from build123d import *

# Parameters (mm, degrees)
SUPPORT_BALISE_W                           = 20
SUPPORT_BALISE_H                           = 350
SUPPORT_BALISE_BOSSAGE_DEPTH               = 80
ESQUISSE3_W                                = 80
ESQUISSE3_H                                = 80
SUPPORT_CHEVAL_ENLEVEMENT_DE_MATIERE_DEPTH = 10
ESQUISSE8_W                                = 10
ESQUISSE8_H                                = 70
SUPPORT_CHEVAL_DEPTH                       = 80
VIS_REACH                                  = 376.466
SERRAGE_VIS_R                              = 2.5
VIS_DIRECTION_2_DEPTH                      = 375.466286867
ENL_V_MAT_EXTRU_5_DEPTH                    = 20
POUR_IMPRESSION_R                          = 15
FIXATION_POUR_ASSEMBLAGE_R                 = 2
VIS_POUR_ASSEMBLAGE_DEPTH                  = 20
ENL_V_MAT_EXTRU_6_DEPTH                    = 378.359245282
ENL_V_MAT_EXTRU_6_DEPTH_BACK               = 378.359245282
PARTIE_HAUTE_W                             = 433.052929697
PARTIE_HAUTE_H                             = 227.316532038


with BuildPart() as part:
    # Support Balise → Support balise bossage (new body)
    with BuildSketch(Plane.XY):
        with Locations((10, 175)):
            Rectangle(SUPPORT_BALISE_W, SUPPORT_BALISE_H)
    extrude(amount=SUPPORT_BALISE_BOSSAGE_DEPTH)

    # Esquisse3 → Support Cheval enlevement de matiere (add)
    with BuildSketch(Plane(origin=(0, 350, 0), x_dir=(1, 0, 0), z_dir=(0, 1, 0))):
        with Locations((-20, -40)):
            Rectangle(ESQUISSE3_W, ESQUISSE3_H)
    extrude(amount=SUPPORT_CHEVAL_ENLEVEMENT_DE_MATIERE_DEPTH)

    # Esquisse8 → Support Cheval (cut)
    with BuildSketch(Plane.XY.offset(80)):
        with Locations((10, 35)):
            Rectangle(ESQUISSE8_W, ESQUISSE8_H)
    extrude(amount=-SUPPORT_CHEVAL_DEPTH, mode=Mode.SUBTRACT)

    # Vis: up to this face of the body (flat: up to its plane)
    vis_end = Plane(part.part.faces().sort_by_distance((0, 175, 40))[0])
    # Serrage vis → Vis (cut, up to the picked face)
    with BuildSketch(Plane(origin=(5, 0, 0), x_dir=(0, 0, -1), z_dir=(1, 0, 0)), mode=Mode.PRIVATE) as vis_sk1:
        with Locations((-70, 11.284552026)):
            Circle(SERRAGE_VIS_R)
    vis_tool1 = split(extrude(vis_sk1.sketch, amount=-VIS_REACH, mode=Mode.PRIVATE), bisect_by=vis_end, keep=Keep.BOTH, mode=Mode.PRIVATE)
    # Serrage vis → Vis (cut, up to the picked face)
    with BuildSketch(Plane(origin=(5, 0, 0), x_dir=(0, 0, -1), z_dir=(1, 0, 0)), mode=Mode.PRIVATE) as vis_sk2:
        with Locations((-70, 53.057184379)):
            Circle(SERRAGE_VIS_R)
    vis_tool2 = split(extrude(vis_sk2.sketch, amount=-VIS_REACH, mode=Mode.PRIVATE), bisect_by=vis_end, keep=Keep.BOTH, mode=Mode.PRIVATE)
    # Serrage vis → Vis (cut, up to the picked face)
    with BuildSketch(Plane(origin=(5, 0, 0), x_dir=(0, 0, -1), z_dir=(1, 0, 0)), mode=Mode.PRIVATE) as vis_sk3:
        with Locations((-10, 53.057184379)):
            Circle(SERRAGE_VIS_R)
    vis_tool3 = split(extrude(vis_sk3.sketch, amount=-VIS_REACH, mode=Mode.PRIVATE), bisect_by=vis_end, keep=Keep.BOTH, mode=Mode.PRIVATE)
    # Serrage vis → Vis (cut, up to the picked face)
    with BuildSketch(Plane(origin=(5, 0, 0), x_dir=(0, 0, -1), z_dir=(1, 0, 0)), mode=Mode.PRIVATE) as vis_sk4:
        with Locations((-10, 11.284552026)):
            Circle(SERRAGE_VIS_R)
    vis_tool4 = split(extrude(vis_sk4.sketch, amount=-VIS_REACH, mode=Mode.PRIVATE), bisect_by=vis_end, keep=Keep.BOTH, mode=Mode.PRIVATE)
    # Serrage vis → Vis (cut, up to the picked face)
    with BuildSketch(Plane(origin=(5, 0, 0), x_dir=(0, 0, -1), z_dir=(1, 0, 0)), mode=Mode.PRIVATE) as vis_sk5:
        with Locations((-40, 32.170868202)):
            Circle(SERRAGE_VIS_R)
    vis_tool5 = split(extrude(vis_sk5.sketch, amount=-VIS_REACH, mode=Mode.PRIVATE), bisect_by=vis_end, keep=Keep.BOTH, mode=Mode.PRIVATE)
    add(vis_tool1.solids().sort_by(Axis((5, 11.284552, 70), (-1, 0, 0)))[0], mode=Mode.SUBTRACT)
    add(vis_tool2.solids().sort_by(Axis((5, 53.057184, 70), (-1, 0, 0)))[0], mode=Mode.SUBTRACT)
    add(vis_tool3.solids().sort_by(Axis((5, 53.057184, 10), (-1, 0, 0)))[0], mode=Mode.SUBTRACT)
    add(vis_tool4.solids().sort_by(Axis((5, 11.284552, 10), (-1, 0, 0)))[0], mode=Mode.SUBTRACT)
    add(vis_tool5.solids().sort_by(Axis((5, 32.170868, 40), (-1, 0, 0)))[0], mode=Mode.SUBTRACT)

    # Serrage vis → Vis direction 2 (cut)
    with BuildSketch(Plane(origin=(5, 0, 0), x_dir=(0, 0, -1), z_dir=(1, 0, 0))):
        with Locations((-70, 11.284552026)):
            Circle(SERRAGE_VIS_R)
        with Locations((-70, 53.057184379)):
            Circle(SERRAGE_VIS_R)
        with Locations((-10, 53.057184379)):
            Circle(SERRAGE_VIS_R)
        with Locations((-10, 11.284552026)):
            Circle(SERRAGE_VIS_R)
        with Locations((-40, 32.170868202)):
            Circle(SERRAGE_VIS_R)
    extrude(amount=VIS_DIRECTION_2_DEPTH, mode=Mode.SUBTRACT)

    # Design → Enlèv. mat.-Extru.5 (cut)
    with BuildSketch(Plane(origin=(20, 0, 0), x_dir=(0, 0, -1), z_dir=(1, 0, 0))):
        Polygon((-55, 315), (-80, 360), (-80, 92.406088827), (-55, 137.406088827), align=None)
        Polygon((0, 92.406088827), (0, 360), (-25, 315), (-25, 137.406088827), align=None)
    extrude(amount=-ENL_V_MAT_EXTRU_5_DEPTH, mode=Mode.SUBTRACT)

    # Pour Impression
    # the kernel refuses this fillet: 15 mm, written as the material it adds along each edge
    with BuildSketch(Plane(origin=(0, 392.780897855, -18.211609919), x_dir=(1, 0, 0), z_dir=(0, -0.8741572761215375, 0.48564293117863266))) as pour_impression_piece_1_section:
        with BuildLine():
            CenterArc((POUR_IMPRESSION_R, -POUR_IMPRESSION_R), POUR_IMPRESSION_R, 90, 90)
            Line((0, -POUR_IMPRESSION_R), (0, 0))
            Line((0, 0), (POUR_IMPRESSION_R, 0))
        make_face()
    pour_impression_piece_1 = extrude(amount=86.439589046, mode=Mode.PRIVATE)
    pour_impression_piece_1 = split(pour_impression_piece_1, bisect_by=Plane(origin=(4.741525676, 350, 2.029382941), z_dir=(0, 1, 0)), keep=Keep.TOP, mode=Mode.PRIVATE)
    pour_impression_piece_1 = split(pour_impression_piece_1, bisect_by=Plane(origin=(4.741525676, 353.652889294, 0), z_dir=(0, 0, 1)), keep=Keep.TOP, mode=Mode.PRIVATE)
    add(pour_impression_piece_1)
    with BuildSketch(Plane(origin=(0, 317.219102145, 56.232834525), x_dir=(1, 0, 0), z_dir=(0, 0.8741572761215377, 0.4856429311786322))) as pour_impression_piece_2_section:
        with BuildLine():
            CenterArc((POUR_IMPRESSION_R, -POUR_IMPRESSION_R), POUR_IMPRESSION_R, 90, 90)
            Line((0, -POUR_IMPRESSION_R), (0, 0))
            Line((0, 0), (POUR_IMPRESSION_R, 0))
        make_face()
    pour_impression_piece_2 = extrude(amount=86.439589046, mode=Mode.PRIVATE)
    pour_impression_piece_2 = split(pour_impression_piece_2, bisect_by=Plane(origin=(4.741525676, 350, 77.970617059), z_dir=(0, 1, 0)), keep=Keep.TOP, mode=Mode.PRIVATE)
    pour_impression_piece_2 = split(pour_impression_piece_2, bisect_by=Plane(origin=(4.741525676, 353.652889294, 80), z_dir=(0, 0, -1)), keep=Keep.TOP, mode=Mode.PRIVATE)
    add(pour_impression_piece_2)

    # Fixation pour assemblage → Vis pour Assemblage (cut)
    with BuildSketch(Plane(origin=(20, 0, 0), x_dir=(0, 0, -1), z_dir=(1, 0, 0))):
        with Locations((-47.5, 195)):
            Circle(FIXATION_POUR_ASSEMBLAGE_R)
        with Locations((-32.5, 195)):
            Circle(FIXATION_POUR_ASSEMBLAGE_R)
        with Locations((-32.5, 175)):
            Circle(FIXATION_POUR_ASSEMBLAGE_R)
        with Locations((-47.5, 175)):
            Circle(FIXATION_POUR_ASSEMBLAGE_R)
    extrude(amount=-VIS_POUR_ASSEMBLAGE_DEPTH, mode=Mode.SUBTRACT)

    # Partie_Haute → Enlèv. mat.-Extru.6 (cut, two sides: drawn at the far end of the back side and taken through both)
    with BuildSketch(Plane(origin=(20, 0, 0), x_dir=(0, 0, -1), z_dir=(1, 0, 0)).offset(-ENL_V_MAT_EXTRU_6_DEPTH_BACK)):
        with Locations((7.967088797, 71.341733981)):
            Rectangle(PARTIE_HAUTE_W, PARTIE_HAUTE_H)
    extrude(amount=ENL_V_MAT_EXTRU_6_DEPTH + ENL_V_MAT_EXTRU_6_DEPTH_BACK, mode=Mode.SUBTRACT)


solid = part.part
Here's how the part is built. I have some questions about the finished solid (model axes, mm). A direction names the side the tool comes from. Round coordinates to 2 decimals unless told otherwise and drop trailing zeros. Write each loop counter-clockwise with the first axis right and the second up, starting at its lowest first coordinate (ties: lowest second). Pieces come first, ordered by that corner, then holes. Notation, with made-up numbers: (-38, -32) -> (-31, -32) arc R24 cw to (-31, 1) -> close; hole circle Ø6 at (62.5, -18.75). An arc over 180 degrees is marked (long way). One line per item, written item: value.
1) We'd pull the mould along Z, two halves only. Please class faces 1 (the face through (20, 291, 41)), 2 (the face through (10.14, 193.226, 31.577)), 3 (the face through (10.335, 354.569, 77.834)): released by +Z, released by -Z, zero draft, split by the parting line, or undercut.
Filled sheet:
face 1: zero draft
face 2: undercut
face 3: released by +Z
2) If I drill on line 1 (Z direction, x = 10, y = 195); line 2 (Y direction, x = 4, z = 47.5); line 3 (Y direction, x = -10, z = 43.5), over which ranges is the centre line in solid material (lowest first)? Write a range as [from, to].
Filled sheet:
line 1: z = [25, 30.5], [34.5, 45.5], [49.5, 55]
line 2: y = [185, 193], [197, 360]
line 3: y = [350, 360]
3) Suppose I cut it at B-B on y = 195. List the corners of the cut face in (x, z) for me, plus the area to 3 significant figures.
Filled sheet:
outline: (0, 25) -> (20, 25) -> (20, 30.5) -> (0, 30.5) -> close; (0, 34.5) -> (20, 34.5) -> (20, 45.5) -> (0, 45.5) -> close; (0, 49.5) -> (20, 49.5) -> (20, 55) -> (0, 55) -> close
area: 440 mm2
4) I'm going to push flat-ended pins straight in: pin 1 Ø3 at (y, z) = (195, 32.5) entering from +X; pin 2 Ø1 at (x, z) = (-33.5, 62) entering from -Y; pin 3 Ø10 at (x, y) = (7.5, 245.5) entering from -Z; pin 4 Ø16 at (x, y) = (14, 273) entering from +Z. Where does each tip first touch, or does it pass through?
Filled sheet:
pin 1: passes through
pin 2: stops at y = 350
pin 3: stops at z = 25
pin 4: stops at z = 55
5) Suppose I cut it at A-A on z = 32.5. List the corners of the cut face in (x, y) for me.
Filled sheet:
outline: (-60, 350) -> (0, 350) -> (0, 197) -> (20, 197) -> (20, 360) -> (-60, 360) -> close; (0, 185) -> (20, 185) -> (20, 193) -> (0, 193) -> close
6) Suppose I cut it at D-D on z = 19.5. List the corners of the cut face in (x, y) for me, plus the area to 3 significant figures.
Filled sheet:
outline: (-60, 350) -> (0, 350) -> (0, 324.9) -> (20, 324.9) -> (20, 360) -> (-60, 360) -> close
area: 1,300 mm2
7) For faces 4 (the face through (0, 266, 40)), 5 (the face through (-22, 355, 80)), 6 (the face through (10, 251, 25)), 7 (the face through (10, 249, 55)), 8 (the face through (-23, 355, 0)), which set-ups out of +Z, -Z, +X, -X, +Y, -Y let a thin tool reach every point of the face, with its end or its side?
Filled sheet:
face 4: +Z, -Z, -X, -Y
face 5: +Z, +X, -X, +Y, -Y
face 6: -Z, +X, -X, -Y
face 7: +Z, +X, -X, -Y
face 8: -Z, +X, -X, +Y, -Y
8) Suppose I cut it at C-C on x = 8. List the corners of the cut face in (y, z) for me, plus the area to 3 significant figures.
Filled sheet:
outline: (185, 25) -> (315, 25) -> (350, 5.56) -> (350, 3.57) -> (356.43, 0) -> (360, 0) -> (360, 80) -> (356.43, 80) -> (350, 76.43) -> (350, 74.44) -> (315, 55) -> (185, 55) -> close; hole circle Ø4 at (195, 32.5); hole circle Ø4 at (195, 47.5)
area: 6,380 mm2
